Work out the finished part from the listing and answer in its coordinate system (mm). Give positions to 0.01 mm unless a question says otherwise; leave off trailing zeros. Order: outer loops, then holes, each group sorted by start corner. A loop starts at its lowest first (then second) coordinate and runs counter-clockwise, first axis right, second up. Notation, with made-up numbers: (-9, 67.5) -> (45, 67.5) arc R36 ccw to (45, 104.5) -> close; hole circle Ø8 at (89.5, -6.75). An arc over 180 degrees is marked (long way). Answer as CSV lines item,"result". Start each with the question number.
1. A cutting plane is placed at B-B (x = 2). State how many separate pieces and enclosed holes the cut face has, then the cut area to 3 significant figures.
2. A cutting plane is placed at C-C (z = 131.5). Give the vertices of the cut face in (x, y) (3 decimals), then the cut area to 3 significant figures.
3. Find the intervals of material crossed by L1, parallel to Y at x = 0.9, z = 110; L2, parallel to Z at x = 2.7, y = -9; L3, parallel to Y at x = 1, z = 99.25, in increasing order.
4. A cutting plane is placed at A-A (z = 0). Give the vertices of the cut face in (x, y) (1 decimal).
5. Flat-ended cylindrical pins translate along their axes: pin 1 (1 mm diameter, centred on x = 1, y = -9.5, fed in from +Z); pin 2 (1.8 mm diameter, centred on y = 23.015, z = 110, fed in from -X); pin 3 (1 mm diameter, centred on x = 1, z = -75, fed in from +Y); pin 4 (1.5 mm diameter, centred on x = 1.5, y = 19.5, fed in from +Z). Find the tip coordinate at first contact, or state that the pin passes through.
6. A cutting plane is placed at D-D (z = -77). Give the vertices of the cut face in (x, y) (3 decimals), then the cut area to 3 significant figures.
from build123d import *

# Parameters (mm, degrees)
SKETCH1_R                = 13.5
SKETCH1_R_2              = 2.65
SKETCH1_R_3              = 11.1125
BOSS_EXTRUDE1_DEPTH      = 3.175
M2_5X0_45_TAPPED_HOLE1_D = 2.05
F_6_CLEARANCE_HOLE1_D    = 3.7973
F_6_32_TAPPED_HOLE1_D    = 2.7051
FILLET1_R                = 10


with BuildPart() as part:
    # Sketch1 → Boss-Extrude1 (new body)
    with BuildSketch(Plane(origin=(0, 0, 0), x_dir=(0, 0, -1), z_dir=(1, 0, 0))):
        with BuildLine():
            ThreePointArc((-81.469314765, 7.5), (-139.5, 0), (-81.469314765, -7.5))
            Line((-81.469314765, -7.5), (-14.260527909, -7.5))
            ThreePointArc((-14.260527909, -7.5), (0, -16.1125), (14.260527909, -7.5))
            Line((14.260527909, -7.5), (100, -7.5))
            ThreePointArc((100, -7.5), (107.5, 0), (100, 7.5))
            Line((100, 7.5), (14.260527909, 7.5))
            ThreePointArc((14.260527909, 7.5), (0, 16.1125), (-14.260527909, 7.5))
            Line((-14.260527909, 7.5), (-81.469314765, 7.5))
        make_face()
        with Locations((-110, 0)):
            Circle(SKETCH1_R, mode=Mode.SUBTRACT)
        with Locations((-99.25, -18.619546181)):
            Circle(SKETCH1_R_2, mode=Mode.SUBTRACT)
        with Locations((-131.5, 0)):
            Circle(SKETCH1_R_2, mode=Mode.SUBTRACT)
        with Locations((-99.25, 18.619546181)):
            Circle(SKETCH1_R_2, mode=Mode.SUBTRACT)
        Circle(SKETCH1_R_3, mode=Mode.SUBTRACT)
    extrude(amount=BOSS_EXTRUDE1_DEPTH)

    # M2.5x0.45 Tapped Hole1 (through all)
    with Locations(Plane(origin=(3.175, 0, 0), x_dir=(0, 0, -1), z_dir=(1, 0, 0))):
        with Locations((-110, -23.015), (-110, 23.015)):
            Hole(M2_5X0_45_TAPPED_HOLE1_D / 2)

    # #6 Clearance Hole1 (through all)
    with Locations(Plane(origin=(3.175, 0, 0), x_dir=(0, 0, -1), z_dir=(1, 0, 0))):
        with Locations((-55, 0)):
            Hole(F_6_CLEARANCE_HOLE1_D / 2)

    # #6-32 Tapped Hole1 (through all)
    with Locations(Plane(origin=(3.175, 0, 0), x_dir=(0, 0, -1), z_dir=(1, 0, 0))):
        with Locations((100, 0)):
            Hole(F_6_32_TAPPED_HOLE1_D / 2)

    # Fillet1
    fillet1_edges = [part.edges().sort_by_distance(p)[0] for p in [
        (1.5875, 7.5, 81.469314765),
        (1.5875, 7.5, 14.260527909),
        (1.5875, 7.5, -14.260527909),
        (1.5875, -7.5, -14.260527909),
        (1.5875, -7.5, 14.260527909),
        (1.5875, -7.5, 81.469314765),
    ]]
    fillet(fillet1_edges, radius=FILLET1_R)


solid = part.part
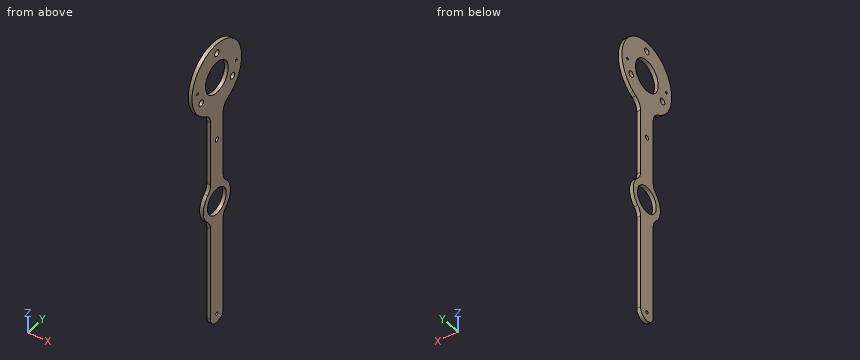
Answer sheet:
1,separate pieces,"1"
1,enclosed holes,"9"
1,area,"4,860 mm^2"
2,outline,"(0, -20.199) -> (3.175, -20.199) -> (3.175, -2.65) -> (0, -2.65) -> close; (0, 2.65) -> (3.175, 2.65) -> (3.175, 20.199) -> (0, 20.199) -> close"
2,area,"111 mm^2"
3,L1,"y = -29.5 to -24.04, -21.99 to -13.5, 13.5 to 21.99, 24.04 to 29.5"
3,L2,"z = -14.11 to -6.52, 6.52 to 14.11, 79.86 to 99.94, 120.06 to 138.09"
3,L3,"y = -27.47 to -21.27, -15.97 to -8.17, 8.17 to 15.97, 21.27 to 27.47"
4,outline,"(0, -16.1) -> (3.2, -16.1) -> (3.2, -11.1) -> (0, -11.1) -> close; (0, 11.1) -> (3.2, 11.1) -> (3.2, 16.1) -> (0, 16.1) -> close"
5,pin 1,"stops at z = 138.09"
5,pin 2,"passes through"
5,pin 3,"stops at y = 7.5"
5,pin 4,"stops at z = 132.77"
6,outline,"(0, -7.5) -> (3.175, -7.5) -> (3.175, 7.5) -> (0, 7.5) -> close"
6,area,"47.6 mm^2"
